Read the model definition and answer for the solid it produces. Units are mm, in the model's axes. Face numbers are marked on the shaded views. Round coordinates to 2 decimals unless told otherwise and drop trailing zeros. Write each loop counter-clockwise with the first axis right and the second up, starting at its lowest first coordinate (ties: lowest second). Pieces come first, ordered by that corner, then holes. Notation, with made-up numbers: (40, 75.25) -> (86, 75.25) arc R23 cw to (86, 91.25) -> close; hole circle Ø5 at (23, -39.5). An arc over 180 degrees is marked (long way). Return JSON: item names as keys, results as strings.
from build123d import *

# Parameters (mm, degrees)
F3_R     = 2
F4_SIZE  = 0.5
F5_R     = 3
F6_DEPTH = 20.001


# Not quite as in the source:
# - a fillet or chamfer that OpenCascade refuses, or shapes differently, is made with other operations: its cross-section is extruded or revolved along the edge and cut away or added


with BuildPart() as f1:
    # F0 (on Front) → F1 (revolve)
    with BuildSketch(Plane.XZ):
        Polygon((0, 20), (0, 0), (25, 0), (25, 10), (21.5, 10), (21.5, 19), (20, 19), (20, 20), align=None)
    revolve(axis=Axis((0, 0, 11.1239180034), (0, 0, -1)))

    # F2: fillet of radius 5 on 1 edges, made by hand

    # F2_s1 → F2_t2 (revolve, cut)
    with BuildSketch(Plane.XZ):
        with BuildLine():
            ThreePointArc((25, 5.2303039929), (24.0311288741, 8.1883438845), (21.5, 10))
            Line((21.5, 10), (25, 10))
            Line((25, 10), (25, 5.2303039929))
        make_face()
    revolve(axis=Axis((0, 0, 10), (0, 0, -1)), mode=Mode.SUBTRACT)

    # F3
    f3_edges = [f1.edges().sort_by_distance(p)[0] for p in [
        (-25, 0, 0),
    ]]
    fillet(f3_edges, radius=F3_R)

    # F4
    f4_edges = [f1.edges().sort_by_distance(p)[0] for p in [
        (-21.5, 0, 19),
        (-20, 0, 19),
    ]]
    chamfer(f4_edges, length=F4_SIZE)

    # F5 (on face) → F6 (cut, through all)
    with BuildSketch(Plane.XY.offset(20)):
        Circle(F5_R)
    extrude(amount=-F6_DEPTH, mode=Mode.SUBTRACT)


solid = f1.part
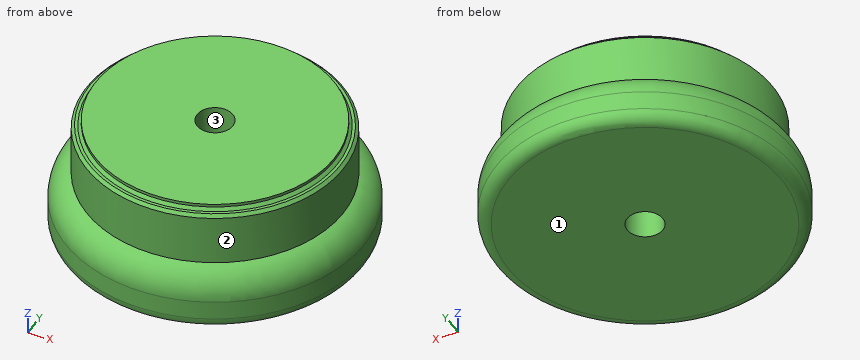
Item 1: Section A-A (x = 0) is taken. Give the vertices of the cut face in (y, z).
Worked answers:
{"outline": "(-25, 2) arc R2 ccw to (-23, 0) -> (-3, 0) -> (-3, 20) -> (-20, 20) -> (-20, 19.5) -> (-20.5, 19) -> (-21, 19) -> (-21.5, 18.5) -> (-21.5, 10) arc R5 ccw to (-25, 5.23) -> close; (3, 0) -> (23, 0) arc R2 ccw to (25, 2) -> (25, 5.23) arc R5 ccw to (21.5, 10) -> (21.5, 18.5) -> (21, 19) -> (20.5, 19) -> (20, 19.5) -> (20, 20) -> (3, 20) -> close"}
Item 2: Flat-ended cylindrical pins translate along their axes: pin 1 (1.5 mm diameter, centred on x = -18.5, z = 2.5, fed in from +Y); pin 2 (10 mm diameter, centred on x = 7, z = 17, fed in from +Y); pin 3 (1 mm diameter, centred on x = -12.5, z = 2.5, fed in from -Y). Find the tip coordinate at first contact, or state that the pin passes through.
Worked answers:
{"pin 1": "stops at y = 17.61", "pin 2": "stops at y = 21.41", "pin 3": "stops at y = -21.93"}
Item 3: Section D-D (z = 7) is taken. Give the vertices of the cut face in (x, y), then the cut area to 3 significant figures.
Worked answers:
{"outline": "circle Ø49.35 at (0, 0); hole circle Ø6 at (0, 0)", "area": "1,880 mm2"}
Item 4: Section C-C (z = 13.5) is taken. Give the vertices of the cut face in (x, y).
Worked answers:
{"outline": "circle Ø43 at (0, 0); hole circle Ø6 at (0, 0)"}
Item 5: Straight lines are drawn through the part: L1, parallel to Y at x = 0, z = 12.5; L2, parallel to Y at x = 0, z = 6.25; L3, parallel to X at y = -9, z = 1.5. For each, find the intervals that lie inside material, in ascending order. Write a range as [from, to].
Worked answers:
{"L1": "y = [-21.5, -3], [3, 21.5]", "L2": "y = [-24.89, -3], [3, 24.89]", "L3": "x = [-23.26, 23.26]"}
Item 6: For a pull along Y with two mould halves and no side action, classify the marked faces 1, 2 and 3 as released by +Y, released by -Y, zero draft, split by the parting line, or undercut.
Worked answers:
{"face 1": "zero draft", "face 2": "split by the parting line", "face 3": "undercut"}
